```python
from build123d import *

# Parameters (mm, degrees)
SKETCH1_R           = 2.286
BOSS_EXTRUDE1_DEPTH = 203.2
SKETCH2_W           = 10.922
SKETCH2_H           = 177.8
CUT_EXTRUDE1_DEPTH  = 11.811
SKETCH3_W           = 6.35
SKETCH3_H           = 177.8
BOSS_EXTRUDE2_DEPTH = 1.27


with BuildPart() as part:
    # Sketch1 → Boss-Extrude1 (new body)
    with BuildSketch(Plane(origin=(0, 0, 0), x_dir=(1, 0, 0), z_dir=(0, 1, 0))):
        with BuildLine():
            Line((38.1, 0), (38.1, 8.209871939))
            Line((38.1, 8.209871939), (8.209871939, 38.1))
            Line((8.209871939, 38.1), (0, 38.1))
            Line((0, 38.1), (0, 34.925))
            Line((0, 34.925), (6.858, 34.925))
            Line((6.858, 34.925), (6.858, 31.75))
            Line((6.858, 31.75), (0, 31.75))
            Line((0, 31.75), (0, 28.575))
            Line((0, 28.575), (8.209871939, 28.575))
            Line((8.209871939, 28.575), (14.530925838, 22.253946102))
            Line((14.530925838, 22.253946102), (10.040797777, 17.763818041))
            ThreePointArc((10.040797777, 17.763818041), (10.040797777, 10.040797777), (17.763818041, 10.040797777))
            Line((17.763818041, 10.040797777), (22.253946102, 14.530925838))
            Line((22.253946102, 14.530925838), (28.575, 8.209871939))
            Line((28.575, 8.209871939), (28.575, 0))
            Line((28.575, 0), (31.75, 0))
            Line((31.75, 0), (31.75, 6.858))
            Line((31.75, 6.858), (34.925, 6.858))
            Line((34.925, 6.858), (34.925, 0))
            Line((34.925, 0), (38.1, 0))
        make_face()
        with Locations(Location((13.902307909, 13.902307909, 0), (0, 0, 270))):
            Circle(SKETCH1_R, mode=Mode.SUBTRACT)
    extrude(amount=BOSS_EXTRUDE1_DEPTH)

    # Sketch2 → Cut-Extrude1 (cut)
    with BuildSketch(Plane(origin=(18.39243597, 0, -18.39243597), x_dir=(0.7071067811865541, 0, 0.7071067811865409), z_dir=(-0.7071067811865409, 0, 0.7071067811865541))):
        with Locations((0, 101.6)):
            Rectangle(SKETCH2_W, SKETCH2_H)
    extrude(amount=CUT_EXTRUDE1_DEPTH, mode=Mode.SUBTRACT)

    # Sketch3 → Boss-Extrude2 (add)
    with BuildSketch(Plane(origin=(18.39243597, 0, -18.39243597), x_dir=(0.7071067811865479, 0, 0.7071067811865472), z_dir=(-0.7071067811865472, 0, 0.7071067811865479))):
        with Locations((0, 101.6)):
            Rectangle(SKETCH3_W, SKETCH3_H)
    extrude(amount=BOSS_EXTRUDE2_DEPTH)


solid = part.part
```
Verification items for the finished model (mm, model axes). A direction names the side the tool comes from. Coordinates: 2 decimals unless noted, no trailing zeros. Order: outer loops, then holes, each group sorted by start corner. A loop starts at its lowest first (then second) coordinate and runs counter-clockwise, first axis right, second up. Notation, with made-up numbers: (-0.5, -7.75) -> (3.5, -7.75) arc R29 ccw to (3.5, 21.25) -> close; hole circle Ø1 at (-22, 70.25). An arc over 180 degrees is marked (long way). Put each result on its own line as item: value. Start each with the question number.
1) Release check for a two-part mould opening along Y. For faces 5 (the flat face through (6.858, 100, -33)), 6 (the flat face through (12.5, 190.5, -16)) record: pulls with the +Y half, pulls with the -Y half, needs draft (parallel to the pull), parting line crosses it, or undercut.
2) Cross-section at A-A (x = 4). Enter the section's corners in (y, z) (3 decimals), plus the area to 3 significant figures.
3) Cross-section at C-C (z = -24). Enter the section's corners in (x, y).
4) Tool access check on faces 1 (the flat face through (33, 100, -6.858)), 2 (the flat face through (3, 100, -34.925)), 3 (the flat face through (17.46, 102.84, -17.53)), 4 (the flat face through (28.575, 100, -4)). Record the directions out of +Z, -Z, +X, -X, +Y, -Y that give a thin tool (end or side, any length) a straight path to the whole face; none if there is none.
5) Material ranges on L1, parallel to X at y = 93, z = -3.5 (3 decimals); L2, parallel to Y at x = 11, z = -11; L3, parallel to X at y = 95.5, z = -8 (3 decimals), recorded low to high.
6) Go/stop test with flat-tipped pins: pin 1 (12 mm diameter, centred on y = 45.5, z = -23, fed in from +X); pin 2 (9 mm diameter, centred on y = 146.5, z = -4, fed in from -X); pin 3 (4 mm diameter, centred on x = 13.9, z = -13.9, fed in from +Y); pin 4 (6.5 mm diameter, centred on x = 5.5, y = 102.5, fed in from +Z). Record where each tip stops, or that it passes through.
Geometry check:
1. face 5: needs draft
1. face 6: undercut
2. outline: (0, -38.1) -> (203.2, -38.1) -> (203.2, -34.925) -> (0, -34.925) -> close; (0, -31.75) -> (203.2, -31.75) -> (203.2, -28.575) -> (0, -28.575) -> close
2. area: 1,290 mm^2
3. outline: (12.78, 0) -> (22.31, 0) -> (22.31, 203.2) -> (12.78, 203.2) -> close
4. face 1: +Z, +Y, -Y
4. face 2: -X, +Y, -Y
4. face 3: +Z, -X
4. face 4: +Z, -X, +Y, -Y
5. L1: x = 28.575 to 31.75, 34.925 to 38.1
5. L2: y = 0 to 12.7, 190.5 to 203.2
5. L3: x = 28.575 to 38.1
6. pin 1: stops at x = 29.31
6. pin 2: stops at x = 28.28
6. pin 3: passes through
6. pin 4: stops at z = -28.03
